Here's the drawing with two shaded views (mm, measured from the low corner). I have some questions. A direction names the side the tool comes from. Coordinates: 2 decimals unless noted, no trailing zeros. Loops run counter-clockwise (first coordinate to the right, second up) from the corner with the lowest first, then second, coordinate; pieces in that order, holes last. Notation, with made-up numbers: (-4.75, 40) -> (26.25, 40) arc R28 ccw to (26.25, 77) -> close; hole circle Ø3 at (-36.5, -3.5). An arc over 180 degrees is marked (long way). Use CSV: the item, a comma, the result in double quotes. Start each with the question number.
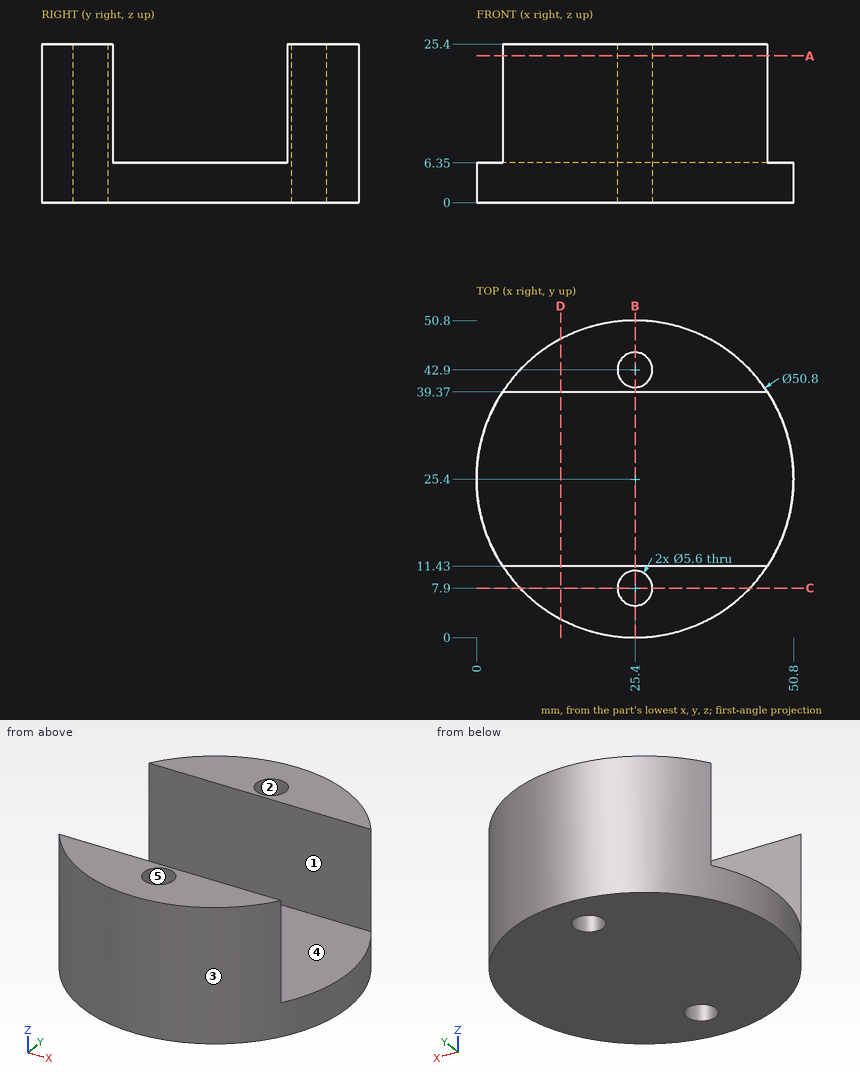
1) I want a section at A-A, the plane z = 23.5. Please give me the cut outline in (x, y), plus the area to 3 significant figures.
2) I want a section at B-B, the plane x = 25.4. Please give me the cut outline in (y, z), plus the area to 3 significant figures.
3) Thinking about a two-plate mould opening in X: for the marked faces 1, 2 and 3, which applies, pulls with the +X half, pulls with the -X half, needs draft (parallel to the pull), parting line crosses it, or undercut?
4) Please list where these lines run through material, in increasing order: L1, parallel to Y at x = 25.4, z = 8; L2, parallel to Y at x = 27, z = 12; L3, parallel to Z at x = 5, y = 14. Write a range as [from, to].
5) I want a section at C-C, the plane y = 7.9. Please give me the cut outline in (x, z).
6) Which directions (+Z, -Z, +X, -X, +Y, -Y) give clear straight access to the entire face, cutting with the end or side of a thin tool? Please do the marked faces 4 and 5.
7) For P1, Ø1.5, axis at x = 8, y = 5.5, coming from the +Z side; P2, Ø3, axis at x = 9.5, z = 10.5, coming from the -Y side; P3, Ø2, axis at y = 10, z = 17.5, coming from the +X side; P4, Ø6, axis at x = 35, y = 34, coming from the +Z side, each with a flat end and sliding along its axis, tell me the tip position at first contact or that it passes through.
8) I want a section at D-D, the plane x = 13.5. Please give me the cut outline in (y, z), plus the area to 3 significant figures.
Return value:
1,outline,"(4.19, 11.43) arc R25.4 ccw to (46.61, 11.43) -> close; (4.19, 39.37) -> (46.61, 39.37) arc R25.4 ccw to start; hole circle Ø5.6 at (25.4, 7.9); hole circle Ø5.6 at (25.4, 42.9)"
1,area,"633 mm²"
2,outline,"(0, 0) -> (5.1, 0) -> (5.1, 25.4) -> (0, 25.4) -> close; (10.7, 0) -> (40.1, 0) -> (40.1, 25.4) -> (39.37, 25.4) -> (39.37, 6.35) -> (11.43, 6.35) -> (11.43, 25.4) -> (10.7, 25.4) -> close; (45.7, 0) -> (50.8, 0) -> (50.8, 25.4) -> (45.7, 25.4) -> close"
2,area,"474 mm²"
3,face 1,"needs draft"
3,face 2,"undercut"
3,face 3,"parting line crosses it"
4,L1,"y = [0, 5.1], [10.7, 11.43], [39.37, 40.1], [45.7, 50.8]"
4,L2,"y = [0.05, 5.6], [10.2, 11.43], [39.37, 40.6], [45.2, 50.75]"
4,L3,"z = [0, 6.35]"
5,outline,"(6.99, 0) -> (22.6, 0) -> (22.6, 25.4) -> (6.99, 25.4) -> close; (28.2, 0) -> (43.81, 0) -> (43.81, 25.4) -> (28.2, 25.4) -> close"
6,face 4,"+Z, +X, -X"
6,face 5,"+Z, -Z"
7,P1,"passes through"
7,P2,"stops at y = 4.48"
7,P3,"stops at x = 46.32"
7,P4,"stops at z = 6.35"
8,outline,"(2.96, 0) -> (47.84, 0) -> (47.84, 25.4) -> (39.37, 25.4) -> (39.37, 6.35) -> (11.43, 6.35) -> (11.43, 25.4) -> (2.96, 25.4) -> close"
8,area,"608 mm²"
